from build123d import *

# Parameters (mm, degrees)
SKETCH1_W          = 1.5
SKETCH1_H          = 2
CUT_EXTRUDE1_DEPTH = 1


with BuildPart() as part:
    # Sketch1 → Revolve1 (revolve)
    with BuildSketch(Plane.XY, mode=Mode.PRIVATE) as revolve1_sk:
        Polygon((0, 3.5), (0, 2), (1.5, 2), (2.75, 2), (2.75, 3.5), align=None)
        with Locations((0.75, 1)):
            Rectangle(SKETCH1_W, SKETCH1_H)
    revolve(revolve1_sk.sketch.rotate(Axis((0, 0, 0), (0, 1, 0)), 90), axis=Axis((0, 0, 0), (0, 1, 0)))

    # Sketch2 → Cut-Extrude1 (cut)
    with BuildSketch(Plane(origin=(0, 3.5, 0), x_dir=(1, 0, 0), z_dir=(0, 1, 0))):
        Polygon((-1.732050808, 0), (-0.866025404, -1.5), (0.866025404, -1.5), (1.732050808, 0), (0.866025404, 1.5), (-0.866025404, 1.5), align=None)
    extrude(amount=-CUT_EXTRUDE1_DEPTH, mode=Mode.SUBTRACT)


solid = part.part
CAD build for the part. Positions are in the model's coordinates, mm. A direction names the side the tool comes from. Give positions to 0.01 mm unless a question says otherwise; leave off trailing zeros. Write each loop counter-clockwise with the first axis right and the second up, starting at its lowest first coordinate (ties: lowest second). Pieces come first, ordered by that corner, then holes. Notation, with made-up numbers: M -19,59.5 L 25,59.5 A23 ccw 25,93.5 Z; hole C 45.5,-28 d2. An arc over 180 degrees is marked long. Put each result on its own line as item: value. Start each with the question number.
(1) Band-saw the part on C-C, the plane z = 0.5. Write the cut outline in (x, y).
(2) Which spindle directions (+Z, -Z, +X, -X, +Y, -Y) get a long thin tool onto all of the face, cutting with end or side? Do faces 5 (the face through (-0.45, 1.01, -1.43)), 6 (the face through (0, 3.5, -2)), 7 (the face through (0, 3, 1.5)). Say none if no direction does.
(3) Band-saw the part on A-A, the plane y = 3.1. Write the cut outline in (x, z).
(4) Band-saw the part on D-D, the plane y = 2.35. Write the cut outline in (x, z).
(5) Band-saw the part on B-B, the plane x = 0. Write the cut outline in (y, z), and give its area (4 significant figures).
(6) Probe L1, parallel to Y at x = 1.15, z = 2.4; L2, parallel to Y at x = -0.6, z = -1; L3, parallel to X at y = 3.2, z = 0.8. List the from-to ranges inside material, lowest first.
(7) Mould opens along X. For faces 1 (the face through (2.685, 2.76, 0.596)), 2 (the face through (-1.293, 3.007, -0.76)), 3 (the face through (0, 0, 0)), 4 (the face through (0, 3, -1.5)) say: +X half, -X half, draft (parallel to the pull), parting line (faces both ways), or undercut.
(8) Flat gauge pins, fed straight in: pin 1 Ø0.9 at (x, z) = (0.5, -0.5) entering from +Y; pin 2 Ø1.5 at (x, y) = (-2, 0.5) entering from -Z; pin 3 Ø1.1 at (x, y) = (-0.5, 3) entering from -Z; pin 4 Ø0.5 at (x, y) = (0.5, 3) entering from +Z. Where does each tip first touch, or does it go through?
Response values:
1. outline: M -2.7,2 L -1.41,2 L -1.41,0 L 1.41,0 L 1.41,2 L 2.7,2 L 2.7,3.5 L 1.44,3.5 L 1.44,2.5 L -1.44,2.5 L -1.44,3.5 L -2.7,3.5 Z
2. face 5: -Y
2. face 6: +Z, -Z, +X, -X, +Y
2. face 7: +Y
3. outline: C 0,0 d5.5; hole M -1.73,0 L -0.87,-1.5 L 0.87,-1.5 L 1.73,0 L 0.87,1.5 L -0.87,1.5 Z
4. outline: C 0,0 d5.5
5. outline: M 0,-1.5 L 2,-1.5 L 2,-2.75 L 3.5,-2.75 L 3.5,-1.5 L 2.5,-1.5 L 2.5,1.5 L 3.5,1.5 L 3.5,2.75 L 2,2.75 L 2,1.5 L 0,1.5 Z
5. area: 11.25 mm2
6. L1: y = 2 to 3.5
6. L2: y = 0 to 2.5
6. L3: x = -2.63 to -1.27, 1.27 to 2.63
7. face 1: parting line
7. face 2: undercut
7. face 3: draft
7. face 4: undercut
8. pin 1: stops at y = 2.5
8. pin 2: stops at z = -0.83
8. pin 3: stops at z = -2.75
8. pin 4: stops at z = 2.74
